Read the model definition and answer for the solid it produces. Units are mm, in the model's axes. Face numbers are marked on the shaded views. A direction names the side the tool comes from. Give positions to 0.01 mm unless a question says otherwise; leave off trailing zeros. Loops run counter-clockwise (first coordinate to the right, second up) from the corner with the lowest first, then second, coordinate; pieces in that order, holes last. Notation, with made-up numbers: M -21,16.25 L 23,16.25 A11 ccw 23,26.25 Z; hole C 81,-20.75 d6. An arc over 180 degrees is marked long. Return JSON: item names as keys, results as strings. Group by question number.
```python
from build123d import *

# Parameters (mm, degrees)
F0_R     = 147.5
F1_DEPTH = 35
F2_R     = 50
F3_DEPTH = 56
F4_R     = 45
F5_DEPTH = 40
F7_DEPTH = 40
F8_R     = 90
F9_DEPTH = 40


with BuildPart() as f1:
    # F0 (on Front) → F1 (new body)
    with BuildSketch(Plane.XZ):
        Circle(F0_R)
    extrude(amount=F1_DEPTH)

    # F2 (on face) → F3 (join)
    with BuildSketch(Plane(origin=(0, 0, 0), x_dir=(-1, 0, 0), z_dir=(0, 1, 0))):
        Circle(F2_R)
    extrude(amount=F3_DEPTH)

    # F4 (on face) → F5 (join)
    with BuildSketch(Plane(origin=(0, 56, 0), x_dir=(-1, 0, 0), z_dir=(0, 1, 0))):
        Circle(F4_R)
    extrude(amount=F5_DEPTH)

    # F6 (on face) → F7 (cut)
    with BuildSketch(Plane.XZ.offset(35)):
        with BuildLine():
            ThreePointArc((36.4554849148, -71.2109375), (0, -80), (-36.4554849148, -71.2109375))
            ThreePointArc((-36.4554849148, -71.2109375), (-4.4254556656, -117.2379556656), (37.5, -80))
            ThreePointArc((37.5, -80), (37.2379556656, -75.5745443344), (36.4554849148, -71.2109375))
        make_face()
        with BuildLine():
            ThreePointArc((36.4554849148, -71.2109375), (0, -42.5), (-36.4554849148, -71.2109375))
            ThreePointArc((-36.4554849148, -71.2109375), (0, -80), (36.4554849148, -71.2109375))
        make_face()
    extrude(amount=-F7_DEPTH, mode=Mode.SUBTRACT)

    # F8 (on Front) → F9 (join)
    with BuildSketch(Plane.XZ):
        Circle(F8_R)
    extrude(amount=-F9_DEPTH)


solid = f1.part
```
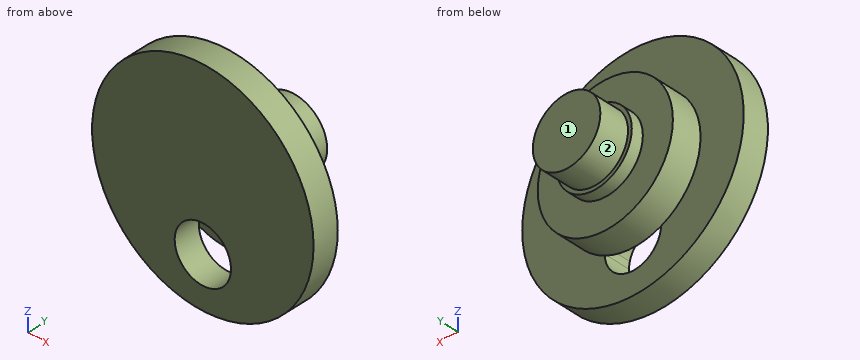
1. Find section C-C (y = -15.5). Write down the section's boundary in (x, z).
2. Find section D-D (x = -74). Write down the section's boundary in (y, z) (3 decimals), and give its area (3 significant figures).
3. Find section B-B (z = 0). Write down the section's boundary in (x, y).
4. Flat-ended cylindrical pins translate along their axes: P1, Ø3, axis at y = 46.5, z = 42, coming from the -X side; P2, Ø5, axis at y = 47.5, z = 16.5, coming from the -X side; P3, Ø5, axis at x = -24.5, y = 23.5, coming from the +Z side. Find the tip coordinate at first contact, or state that the pin passes through.
5. For the marked faces 1 and 2, determine the directions among +Z, -Z, +X, -X, +Y, -Y from which every point of the face is accessible in a straight line to the end or side of a thin tool.
6. Find section A-A (x = 0). Write down the section's boundary in (y, z), and give its area (3 significant figures).
7. Straight lines are drawn through the part: line 1 along Z through (x, y) = (0, -8.5); line 2 along Y through (x, z) = (-88, -35.5); line 3 along X through (y, z) = (-21.5, -80). For each, find the intervals that lie inside material, in ascending order.
Result:
{
 "1": {"outline": "C 0,0 d295; hole C 0,-80 d75"},
 "2": {"outline": "M -35,-127.594 L 0,-127.594 L 0,-51.225 L 40,-51.225 L 40,51.225 L 0,51.225 L 0,127.594 L -35,127.594 Z", "area": "13,000 mm2"},
 "3": {"outline": "M -147.5,-35 L 147.5,-35 L 147.5,0 L 90,0 L 90,40 L 50,40 L 50,56 L 45,56 L 45,96 L -45,96 L -45,56 L -50,56 L -50,40 L -90,40 L -90,0 L -147.5,0 Z"},
 "4": {"P1": "stops at x = -29.32", "P2": "stops at x = -48", "P3": "stops at z = 87.27"},
 "5": {"face 1": "+Z, -Z, +X, -X, +Y", "face 2": "+Y"},
 "6": {"outline": "M -35,-147.5 L 0,-147.5 L 0,-117.5 L -35,-117.5 Z; M -35,-42.5 L 0,-42.5 L 0,-90 L 40,-90 L 40,-50 L 56,-50 L 56,-45 L 96,-45 L 96,45 L 56,45 L 56,50 L 40,50 L 40,90 L 0,90 L 0,147.5 L -35,147.5 Z", "area": "20,100 mm2"},
 "7": {"line 1": "z = -147.5 to -117.5, -42.5 to 147.5", "line 2": "y = -35 to 0", "line 3": "x = -123.92 to -37.5, 37.5 to 123.92"}
}
